Verification items for the finished model (mm, model axes). A direction names the side the tool comes from. Give positions to 0.01 mm unless a question says otherwise; leave off trailing zeros. Write each loop counter-clockwise with the first axis right and the second up, starting at its lowest first coordinate (ties: lowest second). Pieces come first, ordered by that corner, then holes. Notation, with made-up numbers: (27, -37.75) -> (31, -37.75) arc R24 cw to (31, -3.75) -> close; hole circle Ø7 at (26.25, 13.25). An arc over 180 degrees is marked (long way). Answer as CSV lines item,"result".
```python
from build123d import *

# Parameters (mm, degrees)
SKETCH1_W           = 42.57
SKETCH1_H           = 42.57
BOSS_EXTRUDE1_DEPTH = 3
BOSS_EXTRUDE2_DEPTH = 4
SKETCH3_R           = 2.1
CUT_EXTRUDE1_DEPTH  = 2


with BuildPart() as part:
    # Sketch1 → Boss-Extrude1 (new body)
    with BuildSketch(Plane(origin=(0, 0, 0), x_dir=(0, 1, 0), z_dir=(0, 0, 1))):
        Rectangle(SKETCH1_W, SKETCH1_H)
    extrude(amount=BOSS_EXTRUDE1_DEPTH)

    # Sketch2 → Boss-Extrude2 (add)
    with BuildSketch(Plane.XY.offset(3)):
        Polygon((21.285, 21.285), (-21.285, 21.285), (-21.285, -21.285), (-19.285, -21.285), (-19.285, 19.285), (21.285, 19.285), align=None)
    extrude(amount=BOSS_EXTRUDE2_DEPTH)

    # Sketch3 → Cut-Extrude1 (cut)
    with BuildSketch(Plane(origin=(0, 0, 0), x_dir=(1, 0, 0), z_dir=(0, 0, -1))):
        with Locations(Location((-14.213932188, -14.213932188, 0), (0, 0, 180))):
            Circle(SKETCH3_R)
        with Locations(Location((14.213932188, 14.213932188, 0), (0, 0, 180))):
            Circle(SKETCH3_R)
    extrude(amount=-CUT_EXTRUDE1_DEPTH, mode=Mode.SUBTRACT)


solid = part.part
```
1) Draft check along X on faces 1 (the flat face through (-21.285, 0, 3)), 2 (the flat face through (0, 21.285, 3)), 3 (the flat face through (-14, 14, 2)). Enter one of: +X half, -X half, draft (parallel to the pull), parting line (faces both ways), or undercut.
Reported:
face 1,"-X half"
face 2,"draft"
face 3,"undercut"
2) Scan lines: line 1 along Y through (x, z) = (-7, 3.75) (3 decimals); line 2 along Z through (x, y) = (-17.5, 8); line 3 along Y through (x, z) = (14, 1) (3 decimals). Record each from-to range of solid material in increasing order.
Reported:
line 1,"19.285 to 21.285"
line 2,"0 to 3"
line 3,"-21.285 to -16.303, -12.125 to 21.285"
3) Depth check by flat-ended pin: pin 1 (4 mm diameter, centred on x = 14.21, y = -14.21, fed in from -Z); pin 2 (12 mm diameter, centred on x = 13, y = -11, fed in from +Z); pin 3 (2 mm diameter, centred on y = 8.5, z = 4.5, fed in from +X) (3 decimals). Enter the tip coordinate at first touch or a pass-through.
Reported:
pin 1,"z = 2"
pin 2,"z = 3"
pin 3,"x = -19.285"
4) Section check B-B (z = 4.5). Record the boundary of the cut face in (x, y) (3 decimals).
Reported:
outline,"(-21.285, -21.285) -> (-19.285, -21.285) -> (-19.285, 19.285) -> (21.285, 19.285) -> (21.285, 21.285) -> (-21.285, 21.285) -> close"
5) Tool access check on faces 4 (the flat face through (1, 19.285, 5)), 5 (the flat face through (0, 0, 0)), 6 (the cylindrical face through (13.085, -12.443, 0.986)). Record the directions out of +Z, -Z, +X, -X, +Y, -Y that give a thin tool (end or side, any length) a straight path to the whole face; none if there is none.
Reported:
face 4,"+Z, +X, -Y"
face 5,"-Z, +X, -X, +Y, -Y"
face 6,"-Z"
6) Section check C-C (z = 1.5). Record the boundary of the cut face in (x, y) (3 decimals), and give its area (3 significant figures).
Reported:
outline,"(-21.285, -21.285) -> (21.285, -21.285) -> (21.285, 21.285) -> (-21.285, 21.285) -> close; hole circle Ø4.2 at (-14.214, 14.214); hole circle Ø4.2 at (14.214, -14.214)"
area,"1,780 mm²"
7) Section check A-A (y = 0.5). Record the boundary of the cut face in (x, z) (3 decimals), and give its area (3 significant figures).
Reported:
outline,"(-21.285, 0) -> (21.285, 0) -> (21.285, 3) -> (-19.285, 3) -> (-19.285, 7) -> (-21.285, 7) -> close"
area,"136 mm²"
8) Section check D-D (y = 15). Record the boundary of the cut face in (x, z) (3 decimals), and give its area (3 significant figures).
Reported:
outline,"(-21.285, 0) -> (-16.161, 0) -> (-16.161, 2) -> (-12.267, 2) -> (-12.267, 0) -> (21.285, 0) -> (21.285, 3) -> (-19.285, 3) -> (-19.285, 7) -> (-21.285, 7) -> close"
area,"128 mm²"
